Model file for the job. Use its own axes, mm. Face numbers are marked on the shaded views. A direction names the side the tool comes from. Round coordinates to 2 decimals unless told otherwise and drop trailing zeros. Loops run counter-clockwise (first coordinate to the right, second up) from the corner with the lowest first, then second, coordinate; pieces in that order, holes last. Notation, with made-up numbers: M 32.25,-6.75 L 90.25,-6.75 A9 cw 90.25,7.25 Z; hole C 8,-18.75 d7. An arc over 180 degrees is marked long. Use a Markdown table: item, result. Add a question column.
Item 1: Wall check: L1, parallel to Z at x = 3.5, y = -5; L2, parallel to X at y = 18.5, z = 6.5; L3, parallel to X at y = 0, z = 5.5. Give the ranges that are in metal, low to high. Write a range as from..to.
Item 2: Tool access for the marked faces 1, 2 and 3: list every direction of +Z, -Z, +X, -X, +Y, -Y with a clear straight run to the whole face (end or side of a thin tool).
Item 3: Saw through at B-B on y = -12. Write the cut outline in (x, z).
Item 4: Pin check, flat tips, straight feed: P1, Ø10.5, axis at x = -7.5, y = -6, coming from the -Z side (3 decimals); P2, Ø3.5, axis at x = -15, y = 1.5, coming from the -Z side (3 decimals); P3, Ø12, axis at x = 13.5, z = 4, coming from the -Y side. Stop position of each tip, or through.
Item 5: Saw through at C-C on x = 11. Write the cut outline in (y, z), then the cut area to 3 significant figures.
Item 6: Saw through at A-A on z = -13.5. Write the cut outline in (x, y).
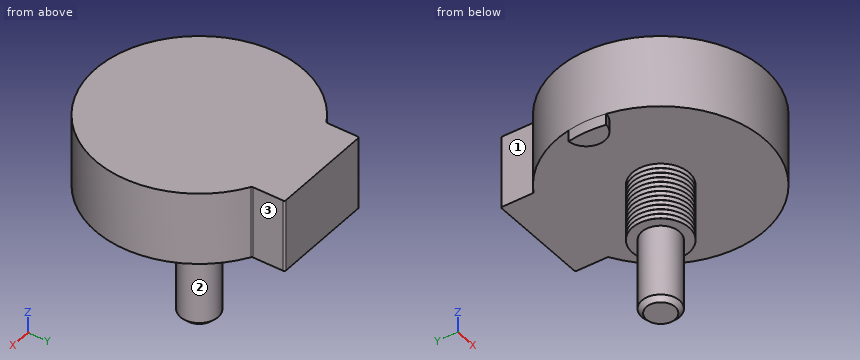
```python
from build123d import *

# Parameters (mm, degrees)
EXTRUDE1_DEPTH      = 12.192
EXTRUDE3_DEPTH      = 1.27
CHAMFER1_SIZE       = 0.762
FILLET1_R           = 0.254
BOSS_EXTRUDE1_START = 1.905
BOSS_EXTRUDE1_DEPTH = 1.905


with BuildPart() as part:
    # Sketch1 → Extrude1 (new body)
    with BuildSketch(Plane.XY):
        with BuildLine():
            Line((-8.73125, 15.122968614), (-8.73125, 20.6375))
            Line((-8.73125, 20.6375), (8.73125, 20.6375))
            Line((8.73125, 20.6375), (8.73125, 15.122968614))
            ThreePointArc((8.73125, 15.122968614), (0, -17.4625), (-8.73125, 15.122968614))
        make_face()
    extrude(amount=EXTRUDE1_DEPTH)



with BuildPart() as body_2:
    # Sketch3 → Extrude3 (new body)
    with BuildSketch(Plane(origin=(0, 0, 0), x_dir=(-1, 0, 0), z_dir=(0, 0, -1))):
        Polygon((3.175, 1.833087105), (0, 3.666174209), (-3.175, 1.833087105), (-3.175, -1.833087105), (0, -3.666174209), (3.175, -1.833087105), align=None)
    extrude(amount=EXTRUDE3_DEPTH)


with BuildPart() as part_1:
    add(part.part)

    add(body_2.part)  # Revolve1 merges body 2
    # Sketch5 → Revolve1 (revolve)
    with BuildSketch(Plane(origin=(0, 0, 0), x_dir=(1, 0, 0), z_dir=(0, 1, 0))):
        Polygon((0, 0), (0, 22.225), (3.16865, 22.225), (3.16865, 9.525), (4.7625, 9.525), (4.318, 9.128125), (4.7625, 8.73125), (4.318, 8.334375), (4.7625, 7.9375), (4.318, 7.540625), (4.7625, 7.14375), (4.318, 6.746875), (4.7625, 6.35), (4.318, 5.953125), (4.7625, 5.55625), (4.318, 5.159375), (4.7625, 4.7625), (4.318, 4.365625), (4.7625, 3.96875), (4.318, 3.571875), (4.7625, 3.175), (4.318, 2.778125), (4.7625, 2.38125), (4.318, 1.984375), (4.7625, 1.5875), (4.318, 1.190625), (4.7625, 0.79375), (4.318, 0.396875), (4.7625, 0), align=None)
    revolve(axis=Axis((0, 0, 0), (0, 0, -1)))

    # Chamfer1
    chamfer1_edges = [part_1.edges().sort_by_distance(p)[0] for p in [
        (-3.16865, 0, -22.225),
    ]]
    chamfer(chamfer1_edges, length=CHAMFER1_SIZE)

    # Fillet1
    fillet1_edges = [part_1.edges().sort_by_distance(p)[0] for p in [
        (-8.73125, 15.122968614, 6.096),
        (-8.73125, 20.6375, 6.096),
        (8.73125, 20.6375, 6.096),
        (8.73125, 15.122968614, 6.096),
    ]]
    fillet(fillet1_edges, radius=FILLET1_R)

    # Sketch6 → Boss-Extrude1 (add)
    with BuildSketch(Plane(origin=(0, 0, 0), x_dir=(-1, 0, 0), z_dir=(0, 0, -1)).offset(BOSS_EXTRUDE1_START)):
        with BuildLine():
            ThreePointArc((17.173863636, 3.161852946), (14.2875, 0), (17.173863636, -3.161852946))
            ThreePointArc((17.173863636, -3.161852946), (17.4625, 0), (17.173863636, 3.161852946))
        make_face()
    extrude(amount=-BOSS_EXTRUDE1_DEPTH)


solid = part_1.part
```
Entries:
| question | item | result |
|---|---|---|
| 1 | L1 | 0..12.19 |
| 1 | L2 | -8.73..8.73 |
| 1 | L3 | -17.46..17.46 |
| 2 | face 1 | +Z, -Z, -X, +Y |
| 2 | face 2 | -Z |
| 2 | face 3 | +Z, -Z, +X, +Y |
| 3 | outline | M -12.69,0 L 12.69,0 L 12.69,12.19 L -12.69,12.19 Z |
| 4 | P1 | z = -9.525 |
| 4 | P2 | z = -1.905 |
| 4 | P3 | y = -15.77 |
| 5 | outline | M -13.56,0 L 13.56,0 L 13.56,12.19 L -13.56,12.19 Z |
| 5 | area | 331 mm2 |
| 6 | outline | C 0,0 d6.34 |
